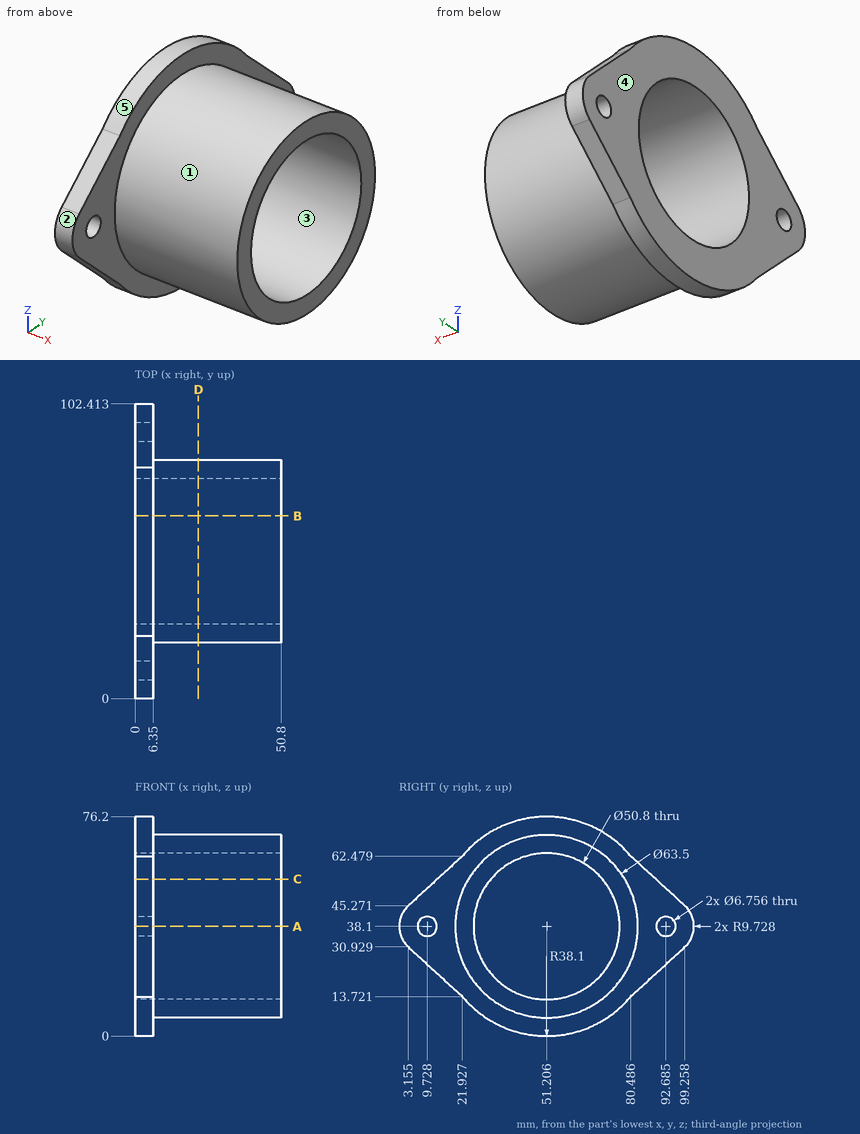
Answer from the drawing. Dimensions are ordinates in mm from the lowest x, y and z of the part. A direction names the side the tool comes from. Round coordinates to 2 decimals unless told otherwise and drop trailing zeros. Loops run counter-clockwise (first coordinate to the right, second up) from the corner with the lowest first, then second, coordinate; pieces in that order, holes last.
(1) The mould has two halves that part along Z. Classify the marked faces 3, 4 and 5: pulls with the +Z half, pulls with the -Z half, needs draft (parallel to the pull), parting line crosses it, or undercut.
Computed values:
face 3: undercut
face 4: needs draft
face 5: pulls with the +Z half
(2) Each of these flat-tipped pins is pushed along its axis until it touches: P1, Ø10, axis at x = 36, z = 17.5, coming from the -Y side; P2, Ø3, axis at x = 15.5, y = 35, coming from the -Z side; P3, Ø6, axis at x = 40.5, y = 24, coming from the -Z side (1 decimal); P4, Ø5, axis at y = 59.5, z = 57.5, coming from the +X side. Where does it stop, or does it pass through?
Computed values:
P1: stops at y = 23.55
P2: stops at z = 9.96
P3: stops at z = 17.6
P4: passes through
(3) The part is cut by section D-D, the plane x = 22. Give the vertices of the cut face in (y, z), and give its area (3 significant figures).
Computed values:
outline: circle Ø63.5 at (51.21, 38.1); hole circle Ø50.8 at (51.21, 38.1)
area: 1,140 mm2
(4) For the marked faces 1 and 2, determine the directions among +Z, -Z, +X, -X, +Y, -Y from which every point of the face is accessible in a straight line to the end or side of a thin tool.
Computed values:
face 1: +X
face 2: +X, -X, -Y
(5) The part is cut by section A-A, the plane z = 38.1. Give the vertices of the cut face in (x, y).
Computed values:
outline: (0, 0) - (6.35, 0) - (6.35, 6.35) - (0, 6.35) - close; (0, 13.11) - (6.35, 13.11) - (6.35, 19.46) - (50.8, 19.46) - (50.8, 25.81) - (0, 25.81) - close; (0, 76.61) - (50.8, 76.61) - (50.8, 82.96) - (6.35, 82.96) - (6.35, 89.31) - (0, 89.31) - close; (0, 96.06) - (6.35, 96.06) - (6.35, 102.41) - (0, 102.41) - close
(6) Find the intervals of material crossed by L1, parallel to Y at x = 15, z = 38; L2, parallel to X at y = 30, z = 63; L3, parallel to Y at x = 10.5, z = 26 (1 decimal), in increasing order.
Computed values:
L1: y = 19.46 to 25.81, 76.61 to 82.96
L2: x = 0 to 6.35
L3: y = 21.9 to 28.9, 73.5 to 80.6
(7) The part is cut by section B-B, the plane y = 63.5. Give the vertices of the cut face in (x, z).
Computed values:
outline: (0, 2.04) - (6.35, 2.04) - (6.35, 8.83) - (50.8, 8.83) - (50.8, 15.87) - (0, 15.87) - close; (0, 60.33) - (50.8, 60.33) - (50.8, 67.37) - (6.35, 67.37) - (6.35, 74.16) - (0, 74.16) - close
(8) The part is cut by section C-C, the plane z = 54.5. Give the vertices of the cut face in (x, y).
Computed values:
outline: (0, 13.22) - (6.35, 13.22) - (6.35, 24.02) - (50.8, 24.02) - (50.8, 31.81) - (0, 31.81) - close; (0, 70.6) - (50.8, 70.6) - (50.8, 78.39) - (6.35, 78.39) - (6.35, 89.19) - (0, 89.19) - close
